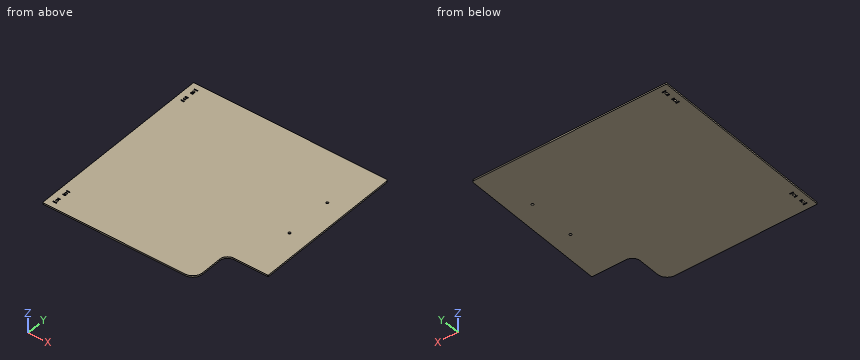
Autodesk Inventor part; units mm, degrees
ref_plane "YZ Plane" through (0, 0, 0) normal (1, 0, 0) x (0, 1, 0)
ref_plane "XZ Plane" through (0, 0, 0) normal (0, 1, 0) x (-1, 0, 0)
ref_plane "XY Plane" through (0, 0, 0) normal (0, 0, 1) x (1, 0, 0)
sketch "Szkic1" plane through (0, 0, 0) normal (0, 0, 1) x (1, 0, 0)
  line L0 (-549.5887, -180.0814) -> (-549.5887, 304.9186)
  line L1 (-549.5887, 304.9186) -> (-53.5887, 304.9186)
  line L2 (-53.5887, 304.9186) -> (-53.5887, -80.0814)
  line L3 (-53.5887, -80.0814) -> (-141.0887, -80.0814)
  line L4 (-161.0887, -100.0814) -> (-161.0887, -155.0814)
  line L5 (-186.0887, -180.0814) -> (-549.5887, -180.0814)
  arc A0 (-141.0887, -80.0814) -> (-161.0887, -100.0814) centre (-141.0887, -100.0814) ccw
  arc A1 (-186.0887, -180.0814) -> (-161.0887, -155.0814) centre (-186.0887, -155.0814) ccw
  point P0 (0, 0)
  point P1 (-161.0887, -80.0814)
  point P2 (-161.0887, -180.0814)
  point P3 (-531.0887, 281.4186)
  point P4 (-531.0887, 253.4186)
  point P5 (-531.0887, -128.5814)
  point P6 (-531.0887, -156.5814)
  point P7 (-103.5887, 173.4186)
  point P8 (-103.5887, 51.4186)
  dimension "d0" = 485
  dimension "d1" = 496
  dimension "d2" = 107.5
  dimension "d3" = 100
  dimension "d6" = 20
  dimension "d7" = 25
  dimension "d8" = 28
  dimension "d9" = 23.5
  dimension "d11" = 28
  dimension "d12" = 23.5
  dimension "d13" = 18.5
  dimension "d14" = 18.5
  dimension "d17" = 18.5
  dimension "d18" = 18.5
  dimension "d31" = 385
  dimension "d32" = 122
  dimension "d33" = 131.5
  dimension "d34" = 50
  dimension "d35" = 50
extrude "Wyciągnięcie proste1" add sketch "Szkic1" along normal blind 4
hole "Otwór1" at (-531.0887, 281.4186, 0) at (-531.0887, 253.4186, 0) at (-531.0887, -128.5814, 0) at (-531.0887, -156.5814, 0) direction (0, 0, 1) diameter 6 end through all
fillet "Zaokrąglenie2" radius 2 2 edges at (-53.5887, -80.0814, 2) (-549.5887, -180.0814, 2)
fillet "Zaokrąglenie2" radius 2 1 edges at (-549.5887, 304.9186, 2)
fillet "Zaokrąglenie2" radius 5 1 edges at (-53.5887, 304.9186, 2)
hole "Otwór2" at (-103.5887, 173.4186, 0) at (-103.5887, 51.4186, 0) direction (0, 0, 1) diameter 6 end through all
sketch "Szkic2" plane through (0, 0, 4) normal (0, 0, 1) x (1, 0, 0)
  circle A0 centre (-103.5887, 173.4186) radius 3
  circle A1 centre (-103.5887, 51.4186) radius 3
  arc A2 (-53.5887, 299.9186) -> (-58.5887, 304.9186) centre (-58.5887, 299.9186) ccw
  line L0 (-58.5887, 304.9186) -> (-547.5887, 304.9186)
  arc A3 (-547.5887, 304.9186) -> (-549.5887, 302.9186) centre (-547.5887, 302.9186) ccw
  line L1 (-549.5887, 302.9186) -> (-549.5887, -178.0814)
  arc A4 (-549.5887, -178.0814) -> (-547.5887, -180.0814) centre (-547.5887, -178.0814) ccw
  line L2 (-547.5887, -180.0814) -> (-186.0887, -180.0814)
  arc A5 (-186.0887, -180.0814) -> (-161.0887, -155.0814) centre (-186.0887, -155.0814) ccw
  line L3 (-161.0887, -155.0814) -> (-161.0887, -100.0814)
  arc A6 (-141.0887, -80.0814) -> (-161.0887, -100.0814) centre (-141.0887, -100.0814) ccw
  line L4 (-141.0887, -80.0814) -> (-55.5887, -80.0814)
  arc A7 (-55.5887, -80.0814) -> (-53.5887, -78.0814) centre (-55.5887, -78.0814) ccw
  line L5 (-53.5887, -78.0814) -> (-53.5887, 299.9186)
  circle A8 centre (-531.0887, -128.5814) radius 3
  circle A9 centre (-531.0887, 281.4186) radius 3
  circle A10 centre (-531.0887, 253.4186) radius 3
  circle A11 centre (-531.0887, -156.5814) radius 3
  line L6 (-535.1387, 289.5186) -> (-527.0387, 289.5186)
  line L7 (-527.0387, 289.5186) -> (-527.0387, 288.1686)
  line L8 (-527.0387, 288.1686) -> (-535.1387, 288.1686)
  line L9 (-535.1387, 288.1686) -> (-535.1387, 289.5186)
  line L10 (-534.1387, 276.1686) -> (-528.0387, 276.1686)
  line L11 (-528.0387, 276.1686) -> (-528.0387, 274.8186)
  line L12 (-528.0387, 274.8186) -> (-534.1387, 274.8186)
  line L13 (-534.1387, 274.8186) -> (-534.1387, 276.1686)
  line L14 (-534.1387, 260.0186) -> (-528.0387, 260.0186)
  line L15 (-528.0387, 260.0186) -> (-528.0387, 258.6686)
  line L16 (-528.0387, 258.6686) -> (-534.1387, 258.6686)
  line L17 (-534.1387, 258.6686) -> (-534.1387, 260.0186)
  line L18 (-535.1387, 245.3186) -> (-527.0387, 245.3186)
  line L19 (-527.0387, 245.3186) -> (-527.0387, 246.6686)
  line L20 (-527.0387, 246.6686) -> (-535.1387, 246.6686)
  line L21 (-535.1387, 246.6686) -> (-535.1387, 245.3186)
  line L22 (-535.6387, 287.6686) -> (-526.5387, 287.6686)
  line L23 (-526.5387, 287.6686) -> (-526.5387, 290.0186)
  line L24 (-526.5387, 290.0186) -> (-535.6387, 290.0186)
  line L25 (-535.6387, 290.0186) -> (-535.6387, 287.6686)
  line L26 (-534.6387, 274.3186) -> (-527.5387, 274.3186)
  line L27 (-527.5387, 274.3186) -> (-527.5387, 276.6686)
  line L28 (-527.5387, 276.6686) -> (-534.6387, 276.6686)
  line L29 (-534.6387, 276.6686) -> (-534.6387, 274.3186)
  line L30 (-534.6387, 258.1686) -> (-527.5387, 258.1686)
  line L31 (-527.5387, 258.1686) -> (-527.5387, 260.5186)
  line L32 (-527.5387, 260.5186) -> (-534.6387, 260.5186)
  line L33 (-534.6387, 260.5186) -> (-534.6387, 258.1686)
  line L34 (-535.6387, 247.1686) -> (-526.5387, 247.1686)
  line L35 (-526.5387, 247.1686) -> (-526.5387, 244.8186)
  line L36 (-526.5387, 244.8186) -> (-535.6387, 244.8186)
  line L37 (-535.6387, 244.8186) -> (-535.6387, 247.1686)
  line L38 (-535.1387, -120.4814) -> (-527.0387, -120.4814)
  line L39 (-527.0387, -120.4814) -> (-527.0387, -121.8314)
  line L40 (-527.0387, -121.8314) -> (-535.1387, -121.8314)
  line L41 (-535.1387, -121.8314) -> (-535.1387, -120.4814)
  line L42 (-534.1387, -133.8314) -> (-528.0387, -133.8314)
  line L43 (-528.0387, -133.8314) -> (-528.0387, -135.1814)
  line L44 (-528.0387, -135.1814) -> (-534.1387, -135.1814)
  line L45 (-534.1387, -135.1814) -> (-534.1387, -133.8314)
  line L46 (-534.1387, -149.9814) -> (-528.0387, -149.9814)
  line L47 (-528.0387, -149.9814) -> (-528.0387, -151.3314)
  line L48 (-528.0387, -151.3314) -> (-534.1387, -151.3314)
  line L49 (-534.1387, -151.3314) -> (-534.1387, -149.9814)
  line L50 (-535.1387, -164.6814) -> (-527.0387, -164.6814)
  line L51 (-527.0387, -164.6814) -> (-527.0387, -163.3314)
  line L52 (-527.0387, -163.3314) -> (-535.1387, -163.3314)
  line L53 (-535.1387, -163.3314) -> (-535.1387, -164.6814)
  line L54 (-535.6387, -122.3314) -> (-526.5387, -122.3314)
  line L55 (-526.5387, -122.3314) -> (-526.5387, -119.9814)
  line L56 (-526.5387, -119.9814) -> (-535.6387, -119.9814)
  line L57 (-535.6387, -119.9814) -> (-535.6387, -122.3314)
  line L58 (-534.6387, -135.6814) -> (-527.5387, -135.6814)
  line L59 (-527.5387, -135.6814) -> (-527.5387, -133.3314)
  line L60 (-527.5387, -133.3314) -> (-534.6387, -133.3314)
  line L61 (-534.6387, -133.3314) -> (-534.6387, -135.6814)
  line L62 (-534.6387, -151.8314) -> (-527.5387, -151.8314)
  line L63 (-527.5387, -151.8314) -> (-527.5387, -149.4814)
  line L64 (-527.5387, -149.4814) -> (-534.6387, -149.4814)
  line L65 (-534.6387, -149.4814) -> (-534.6387, -151.8314)
  line L66 (-535.6387, -162.8314) -> (-526.5387, -162.8314)
  line L67 (-526.5387, -162.8314) -> (-526.5387, -165.1814)
  line L68 (-526.5387, -165.1814) -> (-535.6387, -165.1814)
  line L69 (-535.6387, -165.1814) -> (-535.6387, -162.8314)
  point P0 (0, 0)
  dimension "d43" = 8.1
  dimension "d44" = 1.35
  dimension "d45" = 6.1
  dimension "d46" = 1.35
  dimension "d47" = 6.1
  dimension "d48" = 1.35
  dimension "d49" = 8.1
  dimension "d50" = 1.35
  dimension "d51" = 4.05
  dimension "d52" = 3.05
  dimension "d53" = 3.05
  dimension "d54" = 4.05
  dimension "d55" = 8.1
  dimension "d56" = 8.1
  dimension "d57" = 6.6
  dimension "d59" = 44.2
  dimension "d60" = 17.5
  dimension "d61" = 14.8
  dimension "d62" = 6.6
  dimension "d63" = 0.5
  dimension "d64" = 0.5
  dimension "d65" = 0.5
  dimension "d66" = 0.5
  dimension "d69" = 8.1
  dimension "d70" = 1.35
  dimension "d71" = 6.1
  dimension "d72" = 1.35
  dimension "d73" = 6.1
  dimension "d74" = 1.35
  dimension "d75" = 8.1
  dimension "d76" = 1.35
  dimension "d77" = 44.2
  dimension "d78" = 17.5
  dimension "d79" = 14.8
  dimension "d80" = 0.5
  dimension "d81" = 0.5
  dimension "d82" = 0.5
  dimension "d83" = 0.5
  dimension "d84" = 8.1
  dimension "d85" = 6.6
  dimension "d86" = 6.6
  dimension "d87" = 8.1
  dimension "d88" = 3.05
  dimension "d89" = 4.05
  dimension "d90" = 4.05
  dimension "d91" = 3.05
extrude "Wyciągnięcie proste2" cut sketch "Szkic2" against normal through all contours L6 L7 L8 L9 | L10 L11 L12 L13 | L14 L15 L16 L17 | L21 L20 L19 L18 | L25 L24 L23 L22 | L29 L28 L27 L26 | L33 L32 L31 L30 | L34 L35 L36 L37 | L38 L39 L40 L41 | L42 L43 L44 L45 | L46 L47 L48 L49 | L53 L52 L51 L50 | L57 L56 L55 L54 | L61 L60 L59 L58 | L65 L64 L63 L62 | L66 L67 L68 L69
equation "\"d51\" = 0.5 * d43"
equation "\"d52\" = 0.5 * d45"
equation "\"d53\" = 0.5 * d47"
equation "\"d54\" = 0.5 * d49"
equation "\"d64\" = d63"
equation "\"d65\" = d63"
equation "\"d66\" = d63"
equation "\"d80\" = d63"
equation "\"d81\" = d80"
equation "\"d82\" = d80"
equation "\"d83\" = d80"
properties part number "LC_PLEXI_4mm_Front_Door"
Design review of the part built by this model. Coordinates are the model's own, in mm. Give positions to 0.01 mm unless a question says otherwise; leave off trailing zeros. Loops run counter-clockwise (first coordinate to the right, second up) from the corner with the lowest first, then second, coordinate; pieces in that order, holes last. Notation, with made-up numbers: (85, 56) -> (123, 56) arc R4 ccw to (123, 60) -> close; hole circle Ø1 at (63.5, -23.75). An arc over 180 degrees is marked (long way). One line per question, with ' | ' between items. Start each with the question number.
(1) We need section A-A (z = 2.5). State how many separate pieces and enclosed holes the cut face has, and give its area (3 significant figures).
(2) For line 1 (X direction, y = -151, z = 1.6); line 2 (Y direction, x = -87, z = 1.95); line 3 (X direction, y = 282.5, z = 3), list the stretches that pass through material, from the lowest coordinate up.
(3) Insertion check: P1, Ø1.9, axis at y = -164, z = 2.5, coming from the +X side. The pin has a flat end and moves straight along its axis. Give the tip position at first contact, or say it passes through.
(4) We need section B-B (x = -91). State the section outline as (y, z) points.
The answers:
1) separate pieces: 1 | enclosed holes: 14 | area: 229,000 mm^2
2) line 1: x = -549.59 to -534.64, -527.54 to -161.09 | line 2: y = -80.08 to 304.92 | line 3: x = -549.59 to -533.89, -528.29 to -53.59
3) P1: stops at x = -162.39
4) outline: (-80.08, 0) -> (304.92, 0) -> (304.92, 4) -> (-80.08, 4) -> close
